Check sheet for the modelled part. Datum: model origin and axes. Units: mm. A direction names the side the tool comes from. Round coordinates to 2 decimals unless told otherwise and drop trailing zeros. Order: outer loops, then holes, each group sorted by start corner. A loop starts at its lowest first (then second) coordinate and runs counter-clockwise, first axis right, second up. Notation, with made-up numbers: (48.25, 55.25) -> (92.25, 55.25) arc R33 cw to (92.25, 87.25) -> close; hole circle Ø7 at (-9.5, -8). An arc over 180 degrees is marked (long way). Answer in a Markdown table with one row per item.
Autodesk Inventor part; units mm, degrees
ref_plane "YZ Plane" through (0, 0, 0) normal (1, 0, 0) x (0, 1, 0)
ref_plane "XZ Plane" through (0, 0, 0) normal (0, 1, 0) x (-1, 0, 0)
ref_plane "XY Plane" through (0, 0, 0) normal (0, 0, 1) x (1, 0, 0)
sketch "스케치1" plane through (0, 0, 0) normal (1, 0, 0) x (0, 1, 0)
  line L0 (-15.9064, 9.3186) -> (-7.9064, 9.3186)
  line L1 (-7.9064, 9.3186) -> (-3.9064, 13.3186)
  line L2 (-3.9064, 13.3186) -> (4.0936, 13.3186)
  line L3 (4.0936, 13.3186) -> (8.0936, 9.3186)
  line L4 (8.0936, 9.3186) -> (16.0936, 9.3186)
  line L5 (-15.9064, -1.1814) -> (-16.9064, -2.1814)
  line L6 (-16.9064, -2.1814) -> (-16.9064, -7.1814)
  line L7 (-16.9064, -7.1814) -> (-15.9064, -8.1814)
  line L8 (16.0936, 9.3186) -> (16.0936, -1.1814)
  line L9 (16.0936, -1.1814) -> (17.0936, -2.1814)
  line L10 (17.0936, -2.1814) -> (17.0936, -7.1814)
  line L11 (17.0936, -7.1814) -> (16.0936, -8.1814)
  line L12 (16.0936, -8.1814) -> (-15.9064, -8.1814) construction
  line L13 (-15.9064, -8.6814) -> (16.0936, -8.6814) construction
  line L14 (-15.9064, -8.1814) -> (-15.4064, -8.6814)
  line L15 (-15.4064, -8.6814) -> (-4.4064, -8.6814)
  line L16 (-4.4064, -8.6814) -> (-3.9064, -8.1814)
  line L17 (-3.9064, -8.1814) -> (4.0936, -8.1814)
  line L18 (4.0936, -8.1814) -> (4.5936, -8.6814)
  line L19 (16.0936, -8.1814) -> (15.5936, -8.6814)
  line L20 (15.5936, -8.6814) -> (4.5936, -8.6814)
  line L21 (-11.9064, 9.3186) -> (-11.9064, 8.0705)
  line L22 (16.0936, 8.8186) -> (33.0936, 8.8186)
  line L23 (33.0936, 8.8186) -> (33.0936, -1.1814)
  line L24 (33.0936, -1.1814) -> (16.0936, -1.1814)
  line L25 (17.0936, -1.1814) -> (17.0936, -8.6814)
  line L26 (17.0936, -8.6814) -> (33.0936, -8.6814)
  line L27 (33.0936, -8.6814) -> (33.0936, -1.1814)
  line L28 (-15.9064, 8.8186) -> (-32.9064, 8.8186)
  line L29 (-32.9064, 8.8186) -> (-32.9064, -1.1814)
  line L30 (-32.9064, -1.1814) -> (-15.9064, -1.1814)
  line L31 (-15.9064, -1.1814) -> (-15.9064, 9.3186)
  line L32 (-16.9064, -1.1814) -> (-16.9064, -8.6814)
  line L33 (-16.9064, -8.6814) -> (-32.9064, -8.6814)
  line L34 (-32.9064, -8.6814) -> (-32.9064, -1.1814)
  line L35 (17.0936, -8.6814) -> (15.5936, -8.6814)
  line L36 (-16.9064, -8.6814) -> (-15.4064, -8.6814)
  line L37 (-4.4064, -8.6814) -> (4.5936, -8.6814)
  line L38 (-32.9064, -8.6814) -> (-32.9064, -15.6814)
  line L39 (-32.9064, -15.6814) -> (33.0936, -15.6814)
  line L40 (33.0936, -15.6814) -> (33.0936, -8.6814)
  line L41 (17.0936, -8.6814) -> (17.0936, -15.6814)
  line L42 (-16.9064, -8.6814) -> (-16.9064, -15.6814)
  point P0 (0, 0)
  dimension "d0" = 8
  dimension "d1" = 135
  dimension "d2" = 135
  dimension "d3" = 4
  dimension "d4" = 8
  dimension "d5" = 8
  dimension "d6" = 135
  dimension "d7" = 135
  dimension "d8" = 10.5
  dimension "d10" = 135
  dimension "d11" = 1
  dimension "d12" = 1
  dimension "d13" = 135
  dimension "d14" = 135
  dimension "d15" = 135
  dimension "d16" = 1
  dimension "d17" = 10.5
  dimension "d18" = 5
  dimension "d19" = 5
  dimension "d20" = 0.5
  dimension "d21" = 11
  dimension "d22" = 8
  dimension "d23" = 135
  dimension "d24" = 135
  dimension "d25" = 135
  dimension "d26" = 135
  dimension "d27" = 135
  dimension "d28" = 11
  dimension "d29" = 10
  dimension "d30" = 17
  dimension "d32" = 17
extrude "돌출2" add sketch "스케치1" along normal blind 30 contours L36 L15 L37 L20 L35 L41 L39 L42
sketch "스케치3" plane through (0, -16.9064, -15.6814) normal (0, 0, -1) x (-1, 0, 0)
  line L0 (0, 34) -> (-30, 34)
  line L1 (-30, 0) -> (-30, 34)
  line L2 (-30, 34) -> (-30, 29)
  line L3 (-30, 29) -> (-24, 29)
  circle A0 centre (-24, 29) radius 2.15
  line L4 (-30, 0) -> (-30, 5)
  line L5 (-30, 5) -> (-24, 5)
  circle A1 centre (-24, 5) radius 2.15
  line L6 (0, 34) -> (0, 29)
  line L7 (0, 29) -> (-6, 29)
  circle A2 centre (-6, 29) radius 2.15
  line L8 (0, 0) -> (0, 5)
  line L9 (0, 0) -> (0, 34)
  line L10 (0, 5) -> (-6, 5)
  circle A3 centre (-6, 5) radius 2.15
  line L11 (0, 34) -> (0, 43.5)
  line L12 (-30, 43.5) -> (-30, 34)
  line L13 (-15, 34) -> (-15, 43.5)
  line L14 (-15, 43.5) -> (1, 43.5)
  line L15 (-15, 43.5) -> (-31, 43.5)
  circle A4 centre (1, 43.5) radius 3.8
  circle A5 centre (-31, 43.5) radius 3.8
  line L16 (0, 0) -> (0, -9.5)
  line L17 (-15, -9.5) -> (-15, 0)
  line L18 (-30, -9.5) -> (-30, 0)
  line L19 (-15, -9.5) -> (-31, -9.5)
  line L20 (-15, -9.5) -> (1, -9.5)
  circle A6 centre (-31, -9.5) radius 3.8
  circle A7 centre (1, -9.5) radius 3.8
  point P0 (0, 16.9064)
  dimension "d38" = 5
  dimension "d39" = 6
  dimension "d40" = 4.3
  dimension "d41" = 5
  dimension "d42" = 6
  dimension "d43" = 4.3
  dimension "d44" = 5
  dimension "d45" = 6
  dimension "d46" = 4.3
  dimension "d47" = 5
  dimension "d48" = 6
  dimension "d49" = 4.3
  dimension "d54" = 9.5
  dimension "d55" = 16
  dimension "d56" = 16
  dimension "d57" = 7.6
  dimension "d58" = 7.6
  dimension "d61" = 9.5
  dimension "d62" = 15
  dimension "d67" = 16
  dimension "d68" = 16
  dimension "d69" = 7.6
  dimension "d70" = 7.6
extrude "돌출3" add sketch "스케치1" along normal blind 37 and the other way blind 7 contours L30 L32 L6 L33 L34 | L33 L42 L39 L38 | L41 L26 L40 L39 | L25 L10 L24 L27 L26
extrude "돌출4" cut sketch "스케치3" against normal blind 10 contours A0 | A1 | A3 | A2
extrude "돌출6" cut sketch "스케치3" against normal blind 20 contours A4 L14 L11 | L11 L14 A4 | A5 L15 L12 | L12 L15 A5 | A7 L20 L16 | L16 L20 A7 | A6 L19 L18 | L18 L19 A6
equation "\"d14\" = d13"
equation "\"d15\" = d13"
equation "\"d17\" = d8"
properties part number "xy 조인트"
(1) Section check D-D on y = 24. Record the boundary of the cut face in (x, z), plus the area to 3 significant figures.
Solutions:
| item | result |
|---|---|
| outline | (-7, -15.68) -> (-3.78, -15.68) -> (-3.78, -1.18) -> (-7, -1.18) -> close; (1.78, -15.68) -> (28.22, -15.68) -> (28.22, -1.18) -> (1.78, -1.18) -> close; (33.78, -15.68) -> (37, -15.68) -> (37, -1.18) -> (33.78, -1.18) -> close |
| area | 477 mm^2 |
(2) Section check A-A on x = 31. Record the boundary of the cut face in (y, z).
Solutions:
| item | result |
|---|---|
| outline | (-32.91, -15.68) -> (-30.21, -15.68) -> (-30.21, -1.18) -> (-32.91, -1.18) -> close; (-22.61, -15.68) -> (-16.91, -15.68) -> (-16.91, -1.18) -> (-22.61, -1.18) -> close; (17.09, -15.68) -> (22.79, -15.68) -> (22.79, -1.18) -> (17.09, -1.18) -> close; (30.39, -15.68) -> (33.09, -15.68) -> (33.09, -1.18) -> (30.39, -1.18) -> close |
(3) Tool access check on faces 1 (the cylindrical face through (-0.51, 30.36, -8.53)), 2 (the flat face through (0, 0, -12)). Record the directions out of +Z, -Z, +X, -X, +Y, -Y that give a thin tool (end or side, any length) a straight path to the whole face; none if there is none.
Solutions:
| item | result |
|---|---|
| face 1 | +Z, -Z |
| face 2 | +Z, -Z, -X |
(4) Draft check along Y on faces 3 (the flat face through (15, 0, -8.681)), 4 (the flat face through (15, -32.906, -9)), 5 (the flat face through (37, 25, -8)), 6 (the flat face through (15, 33.094, -9)). Enter one of: pulls with the +Y half, pulls with the -Y half, needs draft (parallel to the pull), parting line crosses it, or undercut.
Solutions:
| item | result |
|---|---|
| face 3 | undercut |
| face 4 | pulls with the -Y half |
| face 5 | needs draft |
| face 6 | pulls with the +Y half |
(5) Depth check by flat-ended pin: pin 1 Ø3 at (x, y) = (4.5, -2.5) entering from +Z; pin 2 Ø1.5 at (y, z) = (-15.5, -9.5) entering from +X; pin 3 Ø2 at (y, z) = (-6.5, -12) entering from -X. Enter the tip coordinate at first touch or a pass-through.
Solutions:
| item | result |
|---|---|
| pin 1 | z = -8.68 |
| pin 2 | x = 30 |
| pin 3 | x = 0 |
(6) Section check C-C on z = -4.25. Record the boundary of the cut face in (x, y).
Solutions:
| item | result |
|---|---|
| outline | (-7, -32.91) -> (37, -32.91) -> (37, -16.91) -> (-7, -16.91) -> close; (-7, 17.09) -> (37, 17.09) -> (37, 33.09) -> (-7, 33.09) -> close; hole circle Ø7.6 at (-1, -26.41); hole circle Ø7.6 at (-1, 26.59); hole circle Ø7.6 at (31, -26.41); hole circle Ø7.6 at (31, 26.59) |
(7) Scan lines: probe 1 along Y at (x, z) = (10.5, -3.5); probe 2 along X at (y, z) = (26.5, -7.5); probe 3 along X at (y, z) = (28.5, -13). Record each from-to range of solid material in increasing order. Write a range as from..to.
Solutions:
| item | result |
|---|---|
| probe 1 | -32.91..-16.91, 17.09..33.09 |
| probe 2 | -7..-4.8, 2.8..27.2, 34.8..37 |
| probe 3 | -7..-4.29, 2.29..27.71, 34.29..37 |
(8) Section check B-B on x = 6. Record the boundary of the cut face in (y, z).
Solutions:
| item | result |
|---|---|
| outline | (-32.91, -15.68) -> (-14.06, -15.68) -> (-14.06, -8.68) -> (-16.91, -8.68) -> (-16.91, -1.18) -> (-32.91, -1.18) -> close; (-9.76, -15.68) -> (9.94, -15.68) -> (9.94, -8.68) -> (-9.76, -8.68) -> close; (14.24, -15.68) -> (33.09, -15.68) -> (33.09, -1.18) -> (17.09, -1.18) -> (17.09, -8.68) -> (14.24, -8.68) -> close |
